Can you work these out from the model? Positions are in its coordinate system, mm. Give positions to 0.01 mm unless a question says otherwise; leave off trailing zeros. Order: outer loops, then holes, each group sorted by start corner. A loop starts at its lowest first (then second) coordinate and runs counter-clockwise, first axis right, second up.
Item 1: If we mould it in two halves opening along Y, with no side actions, what happens to faces 1 (the flat face through (-4, 142, 1.2)), 2 (the conical face through (-0.6, -141.7, 5.7)), 3 (the flat face through (0, 2, 0))? For each: +Y half, -Y half, draft (parallel to the pull), parting line (faces both ways), or undercut.
Item 2: If I drill on line 1 along X through (y, z) = (-106.5, 3); line 2 along X through (y, z) = (111, 1.5); line 3 along Y through (x, z) = (-16, 2.75), over which ranges is the centre line in solid material (lowest first)?
Item 3: I want a section at A-A, the plane y = -97.5. Write out the boundary of the cut face in (x, z).
Item 4: I'm going to push flat-ended pins straight in: pin 1 Ø4.5 at (x, y) = (-28.5, -110) entering from +Z; pin 2 Ø3 at (y, z) = (-102.5, 4) entering from -X. Where does each tip first touch, or does it pass through?
```python
from build123d import *

# Parameters (mm, degrees)
BOSS_EXTRUDE1_DEPTH   = 6
BOSS_EXTRUDE1_TAPER   = 50
F_1_0MM_DOWEL_HOLE2_D = 4
F_4_0MM_DOWEL_HOLE1_D = 4
LPATTERN3_COUNT       = 5
LPATTERN3_PITCH       = 56.5
MIRROR2_COPY_1_D      = 4
MIRROR2_COPY_2_D      = 4
MIRROR2_COPY_3_D      = 4
MIRROR2_COPY_4_D      = 4
SKETCH8_R             = 3.05
CUT_EXTRUDE1_DEPTH    = 4.8


with BuildPart() as part:
    # Sketch1 → Boss-Extrude1 (new body)
    with BuildSketch(Plane.XY):
        with BuildLine():
            ThreePointArc((-32.5, -116), (0, -148.5), (32.5, -116))
            Line((32.5, -116), (32.5, 116))
            ThreePointArc((32.5, 116), (0, 148.5), (-32.5, 116))
            Line((-32.5, 116), (-32.5, -116))
        make_face()
    extrude(amount=BOSS_EXTRUDE1_DEPTH, taper=BOSS_EXTRUDE1_TAPER)

    # Ø1.0mm Dowel Hole2 (through all)
    with Locations(Plane.XY.offset(6)):
        with Locations((-5, 144), (5, 144)):
            f_1_0mm_dowel_hole2 = Hole(F_1_0MM_DOWEL_HOLE2_D / 2)

    # Mirror1: Ø1.0mm Dowel Hole2 across plane
    add(f_1_0mm_dowel_hole2.mirror(Plane.ZX), mode=Mode.SUBTRACT)

    # Ø4.0mm Dowel Hole1 (through all)
    with Locations(Plane.XY.offset(6)):
        with Locations((28.5, 116)):
            f_4_0mm_dowel_hole1 = Hole(F_4_0MM_DOWEL_HOLE1_D / 2)

    # LPattern3: Ø4.0mm Dowel Hole1 ×5
    with Locations(*[(0, -i * LPATTERN3_PITCH, 0) for i in range(1, LPATTERN3_COUNT)]):
        add(f_4_0mm_dowel_hole1, mode=Mode.SUBTRACT)

    # Mirror2: Ø4.0mm Dowel Hole1 across plane
    add(f_4_0mm_dowel_hole1.mirror(Plane(origin=(0, 0, 0), x_dir=(0, 0, 1), z_dir=(1, 0, 0))), mode=Mode.SUBTRACT)

    # Mirror2 copy 1 (through all)
    with Locations(Plane(origin=(0, -56.5, 6), x_dir=(-1, 0, 0), z_dir=(0, 0, 1))):
        with Locations((28.5, -116)):
            Hole(MIRROR2_COPY_1_D / 2)

    # Mirror2 copy 2 (through all)
    with Locations(Plane(origin=(0, -113, 6), x_dir=(-1, 0, 0), z_dir=(0, 0, 1))):
        with Locations((28.5, -116)):
            Hole(MIRROR2_COPY_2_D / 2)

    # Mirror2 copy 3 (through all)
    with Locations(Plane(origin=(0, -169.5, 6), x_dir=(-1, 0, 0), z_dir=(0, 0, 1))):
        with Locations((28.5, -116)):
            Hole(MIRROR2_COPY_3_D / 2)

    # Mirror2 copy 4 (through all)
    with Locations(Plane(origin=(0, -226, 6), x_dir=(-1, 0, 0), z_dir=(0, 0, 1))):
        with Locations((28.5, -116)):
            Hole(MIRROR2_COPY_4_D / 2)

    # Sketch8 → Cut-Extrude1 (cut)
    with BuildSketch(Plane.XY.offset(6)):
        with Locations((-28.5, 116)):
            Circle(SKETCH8_R)
        with Locations((-28.5, 59.5)):
            Circle(SKETCH8_R)
        with Locations((28.5, 59.5)):
            Circle(SKETCH8_R)
        with Locations((28.5, 116)):
            Circle(SKETCH8_R)
        with Locations((28.5, 3)):
            Circle(SKETCH8_R)
        with Locations((-28.5, 3)):
            Circle(SKETCH8_R)
        with Locations((28.5, -53.5)):
            Circle(SKETCH8_R)
        with Locations((-28.5, -53.5)):
            Circle(SKETCH8_R)
        with Locations((-28.5, -110)):
            Circle(SKETCH8_R)
        with Locations((28.5, -110)):
            Circle(SKETCH8_R)
        with Locations((5, -144)):
            Circle(SKETCH8_R)
        with Locations((-5, -144)):
            Circle(SKETCH8_R)
        with Locations((-5, 144)):
            Circle(SKETCH8_R)
        with Locations((5, 144)):
            Circle(SKETCH8_R)
    extrude(amount=-CUT_EXTRUDE1_DEPTH, mode=Mode.SUBTRACT)


solid = part.part
```
Results list:
1. face 1: undercut
1. face 2: -Y half
1. face 3: draft
2. line 1: x = -28.92 to 28.92
2. line 2: x = -30.71 to 30.71
2. line 3: y = -140.45 to 140.45
3. outline: (-32.5, 0) - (32.5, 0) - (25.35, 6) - (-25.35, 6) - close
4. pin 1: stops at z = 1.2
4. pin 2: stops at x = -29.52
